from build123d import *

# Parameters (mm, degrees)
SKETCH1_R           = 31.75
SKETCH1_R_2         = 19.05
BOSS_EXTRUDE1_DEPTH = 12.7
CUT_EXTRUDE1_REACH  = 48.663
SKETCH2_R           = 2.665


with BuildPart() as part:
    # Sketch1 → Boss-Extrude1 (new body)
    with BuildSketch(Plane.XY):
        Circle(SKETCH1_R)
        Circle(SKETCH1_R_2, mode=Mode.SUBTRACT)
    extrude(amount=BOSS_EXTRUDE1_DEPTH)

    # Sketch2 → Cut-Extrude1 (cut, up to next)
    with BuildSketch(Plane.XY.offset(12.7), mode=Mode.PRIVATE) as cut_extrude1_sk1:
        with Locations((0, 25.4)):
            Circle(SKETCH2_R)
    cut_extrude1_tool1 = extrude(cut_extrude1_sk1.sketch, amount=-CUT_EXTRUDE1_REACH, mode=Mode.PRIVATE) & part.part
    # Sketch2 → Cut-Extrude1 (cut, up to next)
    with BuildSketch(Plane.XY.offset(12.7), mode=Mode.PRIVATE) as cut_extrude1_sk2:
        with Locations((21.997045256, 12.7)):
            Circle(SKETCH2_R)
    cut_extrude1_tool2 = extrude(cut_extrude1_sk2.sketch, amount=-CUT_EXTRUDE1_REACH, mode=Mode.PRIVATE) & part.part
    # Sketch2 → Cut-Extrude1 (cut, up to next)
    with BuildSketch(Plane.XY.offset(12.7), mode=Mode.PRIVATE) as cut_extrude1_sk3:
        with Locations((21.997045256, -12.7)):
            Circle(SKETCH2_R)
    cut_extrude1_tool3 = extrude(cut_extrude1_sk3.sketch, amount=-CUT_EXTRUDE1_REACH, mode=Mode.PRIVATE) & part.part
    # Sketch2 → Cut-Extrude1 (cut, up to next)
    with BuildSketch(Plane.XY.offset(12.7), mode=Mode.PRIVATE) as cut_extrude1_sk4:
        with Locations((0, -25.4)):
            Circle(SKETCH2_R)
    cut_extrude1_tool4 = extrude(cut_extrude1_sk4.sketch, amount=-CUT_EXTRUDE1_REACH, mode=Mode.PRIVATE) & part.part
    # Sketch2 → Cut-Extrude1 (cut, up to next)
    with BuildSketch(Plane.XY.offset(12.7), mode=Mode.PRIVATE) as cut_extrude1_sk5:
        with Locations((-21.997045256, -12.7)):
            Circle(SKETCH2_R)
    cut_extrude1_tool5 = extrude(cut_extrude1_sk5.sketch, amount=-CUT_EXTRUDE1_REACH, mode=Mode.PRIVATE) & part.part
    # Sketch2 → Cut-Extrude1 (cut, up to next)
    with BuildSketch(Plane.XY.offset(12.7), mode=Mode.PRIVATE) as cut_extrude1_sk6:
        with Locations((-21.997045256, 12.7)):
            Circle(SKETCH2_R)
    cut_extrude1_tool6 = extrude(cut_extrude1_sk6.sketch, amount=-CUT_EXTRUDE1_REACH, mode=Mode.PRIVATE) & part.part
    add(cut_extrude1_tool1.solids().sort_by_distance((0, 25.4, 12.7))[0], mode=Mode.SUBTRACT)
    add(cut_extrude1_tool2.solids().sort_by_distance((21.997045, 12.7, 12.7))[0], mode=Mode.SUBTRACT)
    add(cut_extrude1_tool3.solids().sort_by_distance((21.997045, -12.7, 12.7))[0], mode=Mode.SUBTRACT)
    add(cut_extrude1_tool4.solids().sort_by_distance((0, -25.4, 12.7))[0], mode=Mode.SUBTRACT)
    add(cut_extrude1_tool5.solids().sort_by_distance((-21.997045, -12.7, 12.7))[0], mode=Mode.SUBTRACT)
    add(cut_extrude1_tool6.solids().sort_by_distance((-21.997045, 12.7, 12.7))[0], mode=Mode.SUBTRACT)


solid = part.part
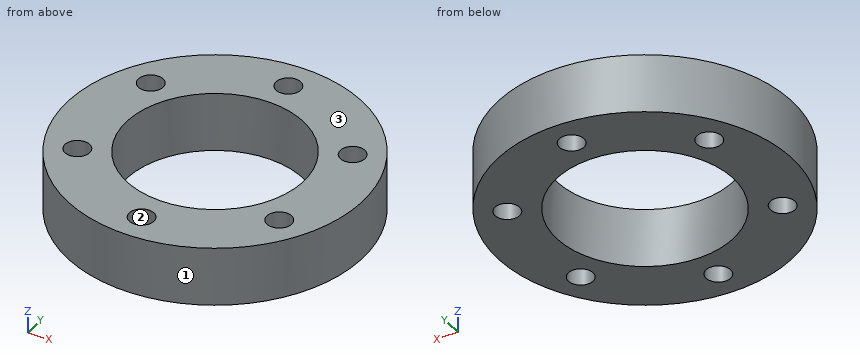
Geometry: final body of the model. Coordinates: model frame, mm. Face numbers are marked on the shaded views. Coordinates: 2 decimals unless noted, no trailing zeros. Order: outer loops, then holes, each group sorted by start corner. A loop starts at its lowest first (then second) coordinate and runs counter-clockwise, first axis right, second up. Notation, with made-up numbers: M -36,-33 L -24,-33 A33 cw -24,-4 Z; hole C 73,81 d10. An arc over 180 degrees is marked long. One line per question, with ' | ' between items. Start each with the question number.
Item 1: Cut plane C-C, the plane z = 6.25. Return the cut outline in (x, y) (3 decimals), then the cut area to 3 significant figures.
Item 2: Cut plane B-B, the plane x = 0. Return the cut outline in (y, z) (3 decimals).
Item 3: Cut plane A-A, the plane y = 0. Return the cut outline in (x, z).
Item 4: Ray query, probe 1 along Y at (x, z) = (0, 7.25) (3 decimals); probe 2 along Y at (x, z) = (-21.5, 11.5); probe 3 along Y at (x, z) = (24, 5.25). Return the intervals inside material, ascending. Write a range as [from, to].
Item 5: Cut plane D-D, the plane y = 25.4. Return the cut outline in (x, z) (3 decimals).
Item 6: Pin query (flat end, axial travel): pin 1 Ø3 at (x, z) = (8.5, 8.5) entering from +Y; pin 2 Ø1 at (y, z) = (6, 5) entering from +X; pin 3 Ø2 at (x, z) = (-1.5, 2.5) entering from +Y. Return the tip coordinate at first contact, or that it passes through.
Item 7: Draft query along Y for the marked faces 1, 2 and 3. Return one class per face: released by +Y, released by -Y, zero draft, split by the parting line, or undercut.
A:
1) outline: C 0,0 d63.5; hole C -21.997,-12.7 d5.33; hole C -21.997,12.7 d5.33; hole C 0,0 d38.1; hole C 0,-25.4 d5.33; hole C 0,25.4 d5.33; hole C 21.997,-12.7 d5.33; hole C 21.997,12.7 d5.33 | area: 1,890 mm2
2) outline: M -31.75,0 L -28.065,0 L -28.065,12.7 L -31.75,12.7 Z; M -22.735,0 L -19.05,0 L -19.05,12.7 L -22.735,12.7 Z; M 19.05,0 L 22.735,0 L 22.735,12.7 L 19.05,12.7 Z; M 28.065,0 L 31.75,0 L 31.75,12.7 L 28.065,12.7 Z
3) outline: M -31.75,0 L -19.05,0 L -19.05,12.7 L -31.75,12.7 Z; M 19.05,0 L 31.75,0 L 31.75,12.7 L 19.05,12.7 Z
4) probe 1: y = [-31.75, -28.065], [-22.735, -19.05], [19.05, 22.735], [28.065, 31.75] | probe 2: y = [-23.36, -15.32], [-10.08, 10.08], [15.32, 23.36] | probe 3: y = [-20.79, -14.46], [-10.94, 10.94], [14.46, 20.79]
5) outline: M -19.05,0 L -2.665,0 L -2.665,12.7 L -19.05,12.7 Z; M 2.665,0 L 19.05,0 L 19.05,12.7 L 2.665,12.7 Z
6) pin 1: stops at y = 30.97 | pin 2: stops at x = 31.27 | pin 3: stops at y = 31.75
7) face 1: split by the parting line | face 2: undercut | face 3: zero draft
